from build123d import *

# Parameters (mm, degrees)
SKETCH1_W           = 100
SKETCH1_H           = 100
BOSS_EXTRUDE1_DEPTH = 3
SKETCH3_W           = 13
SKETCH3_H           = 12
CUT_EXTRUDE3_DEPTH  = 3


with BuildPart() as part:
    # Sketch1 → Boss-Extrude1 (new body)
    with BuildSketch(Plane(origin=(0, 0, 0), x_dir=(1, 0, 0), z_dir=(0, 1, 0))):
        Rectangle(SKETCH1_W, SKETCH1_H)
    extrude(amount=BOSS_EXTRUDE1_DEPTH)

    # Sketch3 → Cut-Extrude3 (cut)
    with BuildSketch(Plane.XZ):
        with Locations((1.5, 27.5)):
            Rectangle(SKETCH3_W, SKETCH3_H)
    extrude(amount=-CUT_EXTRUDE3_DEPTH, mode=Mode.SUBTRACT)


solid = part.part
Geometry check sheet. Reference: the model listing, model coordinates, mm. A direction names the side the tool comes from. Give positions to 0.01 mm unless a question says otherwise; leave off trailing zeros. Write each loop counter-clockwise with the first axis right and the second up, starting at its lowest first coordinate (ties: lowest second). Pieces come first, ordered by that corner, then holes.
1) Cross-section at B-B (z = 24.5). Record the boundary of the cut face in (x, y).
Values follow:
outline: (-50, 0) - (-5, 0) - (-5, 3) - (-50, 3) - close; (8, 0) - (50, 0) - (50, 3) - (8, 3) - close
2) Set-up check for faces 4 (the face through (1, 1, 21.5)), 5 (the face through (-1, 1, -50)): record each of +Z, -Z, +X, -X, +Y, -Y from which the full face is reachable in a straight line by a thin tool's end or side.
Values follow:
face 4: +Y, -Y
face 5: -Z, +X, -X, +Y, -Y
3) Cross-section at A-A (y = 2.4). Record the boundary of the cut face in (x, z), plus the area to 3 significant figures.
Values follow:
outline: (-50, -50) - (50, -50) - (50, 50) - (-50, 50) - close; hole (-5, 21.5) - (8, 21.5) - (8, 33.5) - (-5, 33.5) - close
area: 9,840 mm2
4) Thickness scan on line 1 (X direction, y = 0.4, z = 33). Record the ranges inside material, lowest first.
Values follow:
line 1: x = -50 to -5, 8 to 50
5) Release check for a two-part mould opening along X. For faces 1 (the face through (50, 1, 1)), 2 (the face through (-1, 3, -1)), 3 (the face through (1, 1, 33.5)) record: released by +X, released by -X, zero draft, split by the parting line, or undercut.
Values follow:
face 1: released by +X
face 2: zero draft
face 3: undercut
